Build history of the part. All positions in model axes, mm. Face numbers are marked on the shaded views. A direction names the side the tool comes from. Round coordinates to 2 decimals unless told otherwise and drop trailing zeros. Loops run counter-clockwise (first coordinate to the right, second up) from the corner with the lowest first, then second, coordinate; pieces in that order, holes last. Notation, with made-up numbers: (-16, 7.5) - (15, 7.5) arc R20 cw to (15, 28.5) - close; hole circle Ø7 at (59, 18). An arc over 180 degrees is marked (long way). Put each result on its own line as item: value. Start each with the question number.
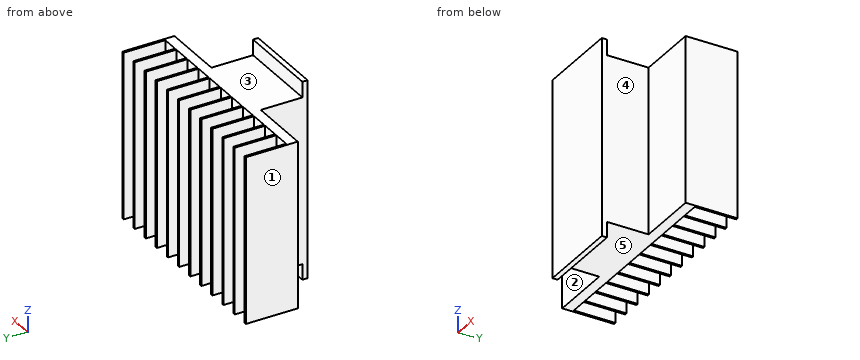
Autodesk Inventor part; units mm, degrees
ref_plane "YZ Plane" through (0, 0, 0) normal (1, 0, 0) x (0, 1, 0)
ref_plane "XZ Plane" through (0, 0, 0) normal (0, 1, 0) x (-1, 0, 0)
ref_plane "XY Plane" through (0, 0, 0) normal (0, 0, 1) x (1, 0, 0)
sketch "Sketch1" plane through (0, 0, 0) normal (0, 1, 0) x (-1, 0, 0)
  line L0 (-63.5, -50.8) -> (63.5, -50.8)
  line L1 (63.5, -50.8) -> (63.5, 50.8)
  line L2 (63.5, 50.8) -> (-63.5, 50.8)
  line L3 (-63.5, 50.8) -> (-63.5, -50.8)
  line L4 (-63.5, -50.8) -> (63.5, 50.8) construction
  line L5 (63.5, -50.8) -> (-63.5, 50.8) construction
  point P0 (0, 0)
  dimension "d0" = 127
  dimension "d1" = 101.6
extrude "Extrusion1" add sketch "Sketch1" along normal blind 31.75
sketch "Sketch2" plane through (-63.5, 0, 50.8) normal (0, 0, 1) x (1, 0, 0)
  line L0 (0, 0) -> (127, 0)
  line L1 (0, 0) -> (0, 6.35)
  line L2 (0, 31.75) -> (127, 31.75)
  line L3 (0, 6.35) -> (127, 6.35) construction
  line L4 (127, 0) -> (0, 0)
  line L5 (0, 6.35) -> (0, 31.75)
  line L6 (0, 31.75) -> (1.27, 31.75)
  line L7 (1.27, 31.75) -> (1.27, 6.35)
  line L8 (1.27, 6.35) -> (0, 6.35)
  line L9 (127, 0) -> (127, 31.75)
  line L10 (127, 31.75) -> (127, 0)
  line L11 (11.43, 6.35) -> (11.43, 31.75)
  line L12 (11.43, 31.75) -> (12.7, 31.75)
  line L13 (12.7, 31.75) -> (12.7, 6.35)
  line L14 (12.7, 6.35) -> (11.43, 6.35)
  line L15 (22.86, 6.35) -> (22.86, 31.75)
  line L16 (22.86, 31.75) -> (24.13, 31.75)
  line L17 (24.13, 31.75) -> (24.13, 6.35)
  line L18 (24.13, 6.35) -> (22.86, 6.35)
  line L19 (34.29, 6.35) -> (34.29, 31.75)
  line L20 (34.29, 31.75) -> (35.56, 31.75)
  line L21 (35.56, 31.75) -> (35.56, 6.35)
  line L22 (35.56, 6.35) -> (34.29, 6.35)
  line L23 (45.72, 6.35) -> (45.72, 31.75)
  line L24 (45.72, 31.75) -> (46.99, 31.75)
  line L25 (46.99, 31.75) -> (46.99, 6.35)
  line L26 (46.99, 6.35) -> (45.72, 6.35)
  line L27 (57.15, 6.35) -> (57.15, 31.75)
  line L28 (57.15, 31.75) -> (58.42, 31.75)
  line L29 (58.42, 31.75) -> (58.42, 6.35)
  line L30 (58.42, 6.35) -> (57.15, 6.35)
  line L31 (68.58, 6.35) -> (68.58, 31.75)
  line L32 (68.58, 31.75) -> (69.85, 31.75)
  line L33 (69.85, 31.75) -> (69.85, 6.35)
  line L34 (69.85, 6.35) -> (68.58, 6.35)
  line L35 (80.01, 6.35) -> (80.01, 31.75)
  line L36 (80.01, 31.75) -> (81.28, 31.75)
  line L37 (81.28, 31.75) -> (81.28, 6.35)
  line L38 (81.28, 6.35) -> (80.01, 6.35)
  line L39 (91.44, 6.35) -> (91.44, 31.75)
  line L40 (91.44, 31.75) -> (92.71, 31.75)
  line L41 (92.71, 31.75) -> (92.71, 6.35)
  line L42 (92.71, 6.35) -> (91.44, 6.35)
  line L43 (102.87, 6.35) -> (102.87, 31.75)
  line L44 (102.87, 31.75) -> (104.14, 31.75)
  line L45 (104.14, 31.75) -> (104.14, 6.35)
  line L46 (104.14, 6.35) -> (102.87, 6.35)
  line L47 (114.3, 6.35) -> (114.3, 31.75)
  line L48 (114.3, 31.75) -> (115.57, 31.75)
  line L49 (115.57, 31.75) -> (115.57, 6.35)
  line L50 (115.57, 6.35) -> (114.3, 6.35)
  line L51 (125.73, 6.35) -> (125.73, 31.75)
  line L52 (125.73, 31.75) -> (127, 31.75)
  line L53 (127, 31.75) -> (127, 6.35)
  line L54 (127, 6.35) -> (125.73, 6.35)
  line L55 (0, 31.75) -> (127, 31.75)
  line L56 (127, 31.75) -> (127, 6.35)
  line L57 (127, 6.35) -> (0, 6.35)
  line L58 (0, 6.35) -> (0, 31.75)
  point P0 (0.635, 31.75)
  point P1 (12.065, 31.75)
  point P2 (23.495, 31.75)
  point P3 (34.925, 31.75)
  point P4 (46.355, 31.75)
  point P5 (57.785, 31.75)
  point P6 (69.215, 31.75)
  point P7 (80.645, 31.75)
  point P8 (92.075, 31.75)
  point P9 (103.505, 31.75)
  point P10 (114.935, 31.75)
  point P11 (126.365, 31.75)
  point P12 (126.365, 31.75)
  point P13 (125.73, 6.35)
  point P14 (115.57, 31.75)
  point P15 (104.14, 6.35)
  point P16 (114.3, 6.35)
  point P17 (114.3, 31.75)
  point P18 (104.14, 31.75)
  point P19 (92.71, 6.35)
  point P20 (102.87, 6.35)
  point P21 (102.87, 31.75)
  point P22 (92.71, 31.75)
  point P23 (81.28, 6.35)
  point P24 (91.44, 6.35)
  point P25 (91.44, 31.75)
  point P26 (81.28, 31.75)
  point P27 (80.01, 6.35)
  point P28 (80.01, 31.75)
  point P29 (69.85, 31.75)
  point P30 (58.42, 6.35)
  point P31 (68.58, 6.35)
  point P32 (68.58, 31.75)
  point P33 (58.42, 31.75)
  point P34 (57.15, 6.35)
  point P35 (57.15, 31.75)
  point P36 (46.99, 31.75)
  point P37 (35.56, 6.35)
  point P38 (45.72, 6.35)
  point P39 (45.72, 31.75)
  point P40 (35.56, 31.75)
  point P41 (24.13, 6.35)
  point P42 (34.29, 31.75)
  point P43 (24.13, 31.75)
  point P44 (12.7, 6.35)
  point P45 (22.86, 31.75)
  point P46 (12.7, 31.75)
  point P47 (11.43, 31.75)
  point P48 (1.27, 31.75)
  dimension "d4" = 6.35
  dimension "d5" = 1.27
  dimension "d36" = 11.43
  dimension "d41" = 0.635
extrude "Extrusion2" cut sketch "Sketch2" against normal blind 122.2375 contours L7 L2 L11 L57 | L57 L49 L2 L51 | L13 L2 L15 L57 | L57 L45 L2 L47 | L17 L2 L19 L57 | L57 L41 L2 L43 | L21 L2 L23 L57 | L57 L37 L2 L39 | L25 L2 L27 L57 | L57 L33 L2 L35 | L29 L2 L31 L57
sketch "Sketch3" plane through (0, 0, 0) normal (0, -1, 0) x (1, 0, 0)
  line L0 (25.4, -60.325) -> (-25.4, -60.325)
  line L1 (-25.4, -60.325) -> (-25.4, 60.325)
  line L2 (-25.4, 60.325) -> (25.4, 60.325)
  line L3 (25.4, 60.325) -> (25.4, -60.325)
  line L4 (25.4, -60.325) -> (-25.4, 60.325) construction
  line L5 (-25.4, -60.325) -> (25.4, 60.325) construction
  point P0 (0, 0)
  dimension "d44" = 50.8
  dimension "d45" = 120.65
extrude "Extrusion3" add sketch "Sketch3" along normal blind 28.575
sketch "Sketch4" plane through (0, 0, 0) normal (0, 1, 0) x (1, 0, 0)
  line L0 (25.4, 50.8) -> (-25.4, 50.8)
  line L1 (25.4, 60.325) -> (25.4, 50.8)
  line L2 (-25.4, 60.325) -> (25.4, 60.325)
  line L3 (-25.4, 50.8) -> (-25.4, 60.325)
  line L4 (-25.4, -50.8) -> (25.4, -50.8)
  line L5 (-25.4, -60.325) -> (-25.4, -50.8)
  line L6 (25.4, -60.325) -> (-25.4, -60.325)
  line L7 (25.4, -50.8) -> (25.4, -60.325)
  line L8 (-25.4, -60.325) -> (-25.4, 60.325)
  line L9 (-25.4, 60.325) -> (25.4, 60.325)
  line L10 (25.4, 60.325) -> (25.4, 50.8)
  line L11 (25.4, 50.8) -> (-25.4, 50.8)
  line L12 (-25.4, 50.8) -> (-25.4, 60.325)
  line L13 (-25.4, -50.8) -> (25.4, -50.8)
  line L14 (25.4, -50.8) -> (25.4, -60.325)
  line L15 (25.4, -60.325) -> (-25.4, -60.325)
  line L16 (-25.4, -60.325) -> (-25.4, -50.8)
  point P0 (0, 0)
extrude "Extrusion4" cut sketch "Sketch4" against normal blind 25.4
properties part number "Heatsink_and_Amplifier"
1) Drop flat-ended pins along their axis: pin 1 Ø3 at (x, z) = (-46.5, 19.5) entering from +Y; pin 2 Ø3 at (x, y) = (5.5, -8) entering from +Z; pin 3 Ø1.5 at (x, y) = (-16.5, -15) entering from -Z. Give the stop position or say it passes through.
2) Drill centre lines: line 1 (Y direction, x = -25.5, z = 39); line 2 (Z direction, x = -33, y = 2.5); line 3 (X direction, y = -2.5, z = 5.5). Where is each one in solid material? Low to high. Write a range as [from, to].
3) Slice it at D-D, the plane x = 48.5. Write the cut outline in (y, z).
4) Slice it at A-A, the plane y = 11. State how many separate pieces and enclosed holes the cut face has, and give its area (3 significant figures).
5) Slice it at B-B, the plane x = -20.5. Write the cut outline in (y, z) (3 decimals), and give its area (3 significant figures).
6) Slice it at C-C, the plane y = -7.5. Write the cut outline in (x, z).
7) Which spindle directions (+Z, -Z, +X, -X, +Y, -Y) get a long thin tool onto all of the face, cutting with end or side? Do the marked faces 1, 2, 3, 4 and 5. Say none if no direction does.
Taken from the geometry:
1. pin 1: stops at y = 6.35
1. pin 2: stops at z = 50.8
1. pin 3: stops at z = -50.8
2. line 1: y = [0, 6.35]
2. line 2: z = [-50.8, 50.8]
2. line 3: x = [-25.4, 25.4]
3. outline: (0, -50.8) - (6.35, -50.8) - (6.35, 50.8) - (0, 50.8) - close
4. separate pieces: 12
4. enclosed holes: 0
4. area: 1,550 mm2
5. outline: (-28.575, -60.325) - (-25.4, -60.325) - (-25.4, -50.8) - (6.35, -50.8) - (6.35, 50.8) - (-25.4, 50.8) - (-25.4, 60.325) - (-28.575, 60.325) - close
5. area: 3,610 mm2
6. outline: (-25.4, -50.8) - (25.4, -50.8) - (25.4, 50.8) - (-25.4, 50.8) - close
7. face 1: +Z, -Z, -X, +Y, -Y
7. face 2: +Z, -Z, -X, -Y
7. face 3: +Z, +X, -X, +Y
7. face 4: +Z, -Z, +X, -Y
7. face 5: -Z, +X, -X, +Y
